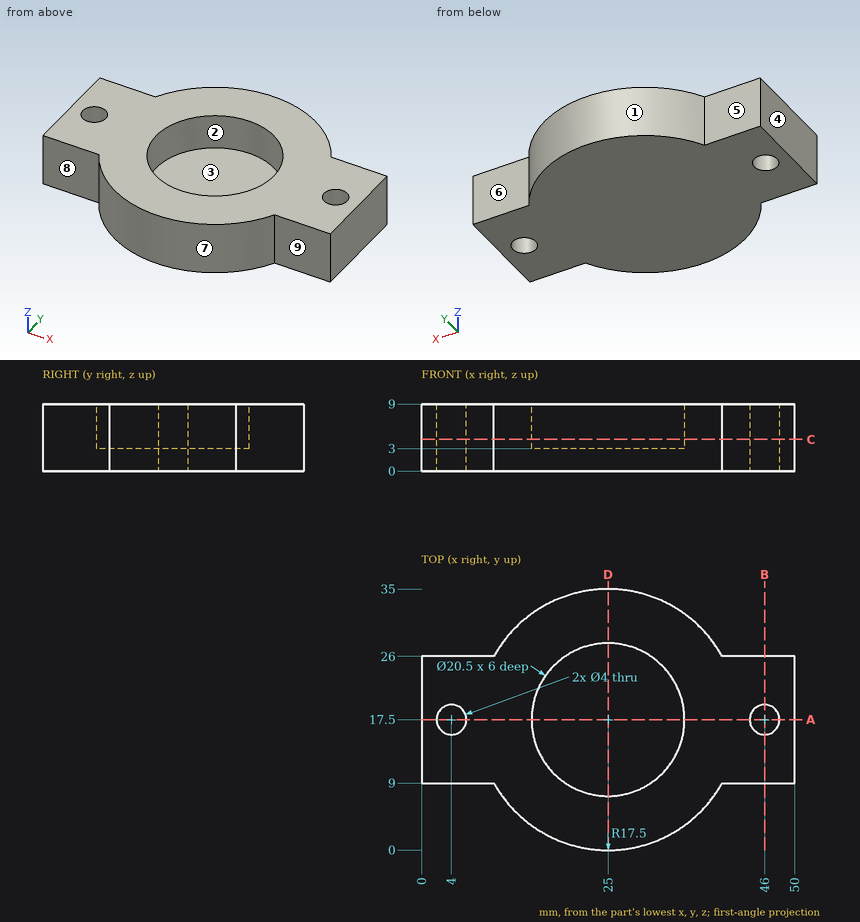
Here's the drawing with two shaded views (mm, measured from the low corner). I have some questions. A direction names the side the tool comes from. Round coordinates to 2 decimals unless told otherwise and drop trailing zeros. Loops run counter-clockwise (first coordinate to the right, second up) from the corner with the lowest first, then second, coordinate; pieces in that order, holes last.
Item 1: Suppose I cut it at B-B, the plane x = 46. Write out the boundary of the cut face in (y, z).
Item 2: Suppose I cut it at C-C, the plane z = 4.25. Write out the boundary of the cut face in (x, y), then the cut area to 3 significant figures.
Item 3: Suppose I cut it at A-A, the plane y = 17.5. Write out the boundary of the cut face in (x, z).
Item 4: Which directions (+Z, -Z, +X, -X, +Y, -Y) give clear straight access to the entire face, cutting with the end or side of a thin tool? Please do the marked faces 5, 6, 7, 8 and 9.
Item 5: If we mould it in two halves opening along X, with no side actions, what happens to the marked faces 1, 2, 3 and 4? For each: +X half, -X half, draft (parallel to the pull), parting line (faces both ways), or undercut.
Item 6: Please list where these lines run through material, in increasing order: L1, parallel to Y at x = 25, z = 6.6; L2, parallel to Y at x = 4, z = 4.75; L3, parallel to X at y = 16, z = 1.5.
Item 7: Will these pins go through, and if not, where does the flat tip stop? pin 1 Ø2 at (x, z) = (26.5, 4) entering from +Y; pin 2 Ø4.5 at (x, z) = (43.5, 2.5) entering from +Y; pin 3 Ø4.5 at (x, z) = (44, 2.5) entering from -Y.
Item 8: Suppose I cut it at D-D, the plane x = 25. Write out the boundary of the cut face in (y, z), then the cut area to 3 significant figures.
Reported:
1. outline: (9, 0) - (15.5, 0) - (15.5, 9) - (9, 9) - close; (19.5, 0) - (26, 0) - (26, 9) - (19.5, 9) - close
2. outline: (0, 9) - (9.7, 9) arc R17.5 ccw to (40.3, 9) - (50, 9) - (50, 26) - (40.3, 26) arc R17.5 ccw to (9.7, 26) - (0, 26) - close; hole circle Ø4 at (4, 17.5); hole circle Ø20.5 at (25, 17.5); hole circle Ø4 at (46, 17.5)
2. area: 886 mm2
3. outline: (0, 0) - (2, 0) - (2, 9) - (0, 9) - close; (6, 0) - (44, 0) - (44, 9) - (35.25, 9) - (35.25, 3) - (14.75, 3) - (14.75, 9) - (6, 9) - close; (48, 0) - (50, 0) - (50, 9) - (48, 9) - close
4. face 5: +Z, -Z, -X, +Y
4. face 6: +Z, -Z, +X, +Y
4. face 7: +Z, -Z, -Y
4. face 8: +Z, -Z, -X, -Y
4. face 9: +Z, -Z, +X, -Y
5. face 1: parting line
5. face 2: undercut
5. face 3: undercut
5. face 4: -X half
6. L1: y = 0 to 7.25, 27.75 to 35
6. L2: y = 9 to 15.5, 19.5 to 26
6. L3: x = 0 to 2.68, 5.32 to 44.68, 47.32 to 50
7. pin 1: stops at y = 34.99
7. pin 2: stops at y = 26
7. pin 3: stops at y = 9
8. outline: (0, 0) - (35, 0) - (35, 9) - (27.75, 9) - (27.75, 3) - (7.25, 3) - (7.25, 9) - (0, 9) - close
8. area: 192 mm2
